Geometry: final body of the model. Coordinates: model frame, mm. Round coordinates to 2 decimals unless told otherwise and drop trailing zeros. Loops run counter-clockwise (first coordinate to the right, second up) from the corner with the lowest first, then second, coordinate; pieces in that order, holes last. Notation, with made-up numbers: (44, 30) - (96, 30) arc R23 ccw to (96, 50) - close; hole circle Ø4 at (-9, -6). An arc over 180 degrees is marked (long way). Write item = value, one per line. Start each with the question number.
Item 1: Section A-A (x = -284). Return loops of the section in (y, z).
Item 2: Section B-B (y = -31.5). Return loops of the section in (x, z), plus the area to 3 significant figures.
Item 3: Line query: line 1 (X direction, y = 23, z = 1.9); line 2 (X direction, y = 266, z = 0.6); line 3 (Y direction, x = -251.5, z = 2.1). Output: solid intervals per line, ascending. Write a range as from..to.
Item 4: First-contact query: pin 1 (1 mm diameter, centred on x = -248.5, z = 4, fed in from +Y) (3 decimals); pin 2 (3 mm diameter, centred on y = 188, z = 2.5, fed in from -X). Flat tips, straight axial feed; report the tip coordinate or a pass-through.
Item 5: Section C-C (z = 2.7). Return loops of the section in (x, y).
from build123d import *

# Parameters (mm, degrees)
F1_DEPTH = 6


with BuildPart() as f1:
    # F0 (on Top) → F1 (new body)
    with BuildSketch(Plane.XY):
        with BuildLine():
            Line((4.290289, -108.624975), (4.290289, 306.075025))
            ThreePointArc((4.290289, 306.075025), (-3.509711, 313.875025), (-11.309711, 306.075025))
            Line((-11.309711, 306.075025), (-11.309711, 96.725025))
            ThreePointArc((-11.309711, 96.725025), (-12.832756, 93.04807), (-16.509711, 91.525025))
            Line((-16.509711, 91.525025), (-441.135317, 91.525025))
            Line((-441.135317, 91.525025), (-461.209711, 91.525025))
            ThreePointArc((-461.209711, 91.525025), (-466.725144, 89.240458), (-469.009711, 83.725025))
            Line((-469.009711, 83.725025), (-469.009711, -108.624975))
            ThreePointArc((-469.009711, -108.624975), (-466.725144, -114.140408), (-461.209711, -116.424975))
            Line((-461.209711, -116.424975), (-3.509711, -116.424975))
            ThreePointArc((-3.509711, -116.424975), (2.005722, -114.140408), (4.290289, -108.624975))
        make_face()
        with BuildLine():
            ThreePointArc((-10.009711, 306.075025), (-3.509711, 312.575025), (2.990289, 306.075025))
            Line((2.990289, 306.075025), (2.990289, -108.624975))
            ThreePointArc((2.990289, -108.624975), (1.086483, -113.221169), (-3.509711, -115.124975))
            Line((-3.509711, -115.124975), (-461.209711, -115.124975))
            ThreePointArc((-461.209711, -115.124975), (-465.805905, -113.221169), (-467.709711, -108.624975))
            Line((-467.709711, -108.624975), (-467.709711, 83.725025))
            ThreePointArc((-467.709711, 83.725025), (-465.805905, 88.321219), (-461.209711, 90.225025))
            Line((-461.209711, 90.225025), (-244.859711, 90.225025))
            Line((-244.859711, 90.225025), (-16.509711, 90.225025))
            ThreePointArc((-16.509711, 90.225025), (-11.913517, 92.128831), (-10.009711, 96.725025))
            Line((-10.009711, 96.725025), (-10.009711, 306.075025))
        make_face(mode=Mode.SUBTRACT)
    extrude(amount=F1_DEPTH)


solid = f1.part
Taken from the geometry:
q1.outline = (-116.42, 0) - (-115.12, 0) - (-115.12, 6) - (-116.42, 6) - close; (90.23, 0) - (91.53, 0) - (91.53, 6) - (90.23, 6) - close
q2.outline = (-469.01, 0) - (-467.71, 0) - (-467.71, 6) - (-469.01, 6) - close; (2.99, 0) - (4.29, 0) - (4.29, 6) - (2.99, 6) - close
q2.area = 15.6 mm^2
q3.line_1 = -469.01..-467.71, 2.99..4.29
q3.line_2 = -11.31..-10.01, 2.99..4.29
q3.line_3 = -116.42..-115.12, 90.23..91.53
q4.pin_1 = 91.525
q4.pin_2 = -11.31
q5.outline = (-469.01, -108.62) arc R7.8 ccw to (-461.21, -116.42) - (-3.51, -116.42) arc R7.8 ccw to (4.29, -108.62) - (4.29, 306.08) arc R7.8 ccw to (-11.31, 306.08) - (-11.31, 96.73) arc R5.2 cw to (-16.51, 91.53) - (-461.21, 91.53) arc R7.8 ccw to (-469.01, 83.73) - close; hole (-467.71, -108.62) arc R6.5 ccw to (-461.21, -115.12) - (-3.51, -115.12) arc R6.5 ccw to (2.99, -108.62) - (2.99, 306.08) arc R6.5 ccw to (-10.01, 306.08) - (-10.01, 96.73) arc R6.5 cw to (-16.51, 90.23) - (-461.21, 90.23) arc R6.5 ccw to (-467.71, 83.73) - close
